```python
from build123d import *

# Parameters (mm, degrees)
SKETCH_R  = 1.05
SKETCH_W  = 12.4
SKETCH_H  = 23
PAD_DEPTH = 3
FILLET_R  = 4


with BuildPart() as part:
    # Sketch → Pad (new body)
    with BuildSketch(Plane.XY):
        Polygon((13, -50), (13, -74), (-13, -74), (-13, -50), (-13, -20), (-13, 12), (13, 12), (13, -20), align=None)
        with Locations((0, -41.76)):
            Circle(SKETCH_R, mode=Mode.SUBTRACT)
        with Locations((0, -69)):
            Circle(SKETCH_R, mode=Mode.SUBTRACT)
        with Locations((0, -55.38)):
            Rectangle(SKETCH_W, SKETCH_H, mode=Mode.SUBTRACT)
        with BuildLine():
            ThreePointArc((-6.5, 6), (-8, 7.5), (-9.5, 6))
            Line((-9.5, 6), (-9.5, -14))
            ThreePointArc((-9.5, -14), (-8, -15.5), (-6.5, -14))
            Line((-6.5, 6), (-6.5, -14))
        make_face(mode=Mode.SUBTRACT)
        with BuildLine():
            ThreePointArc((9.5, 6), (8, 7.5), (6.5, 6))
            Line((6.5, 6), (6.5, -14))
            ThreePointArc((6.5, -14), (8, -15.5), (9.5, -14))
            Line((9.5, 6), (9.5, -14))
        make_face(mode=Mode.SUBTRACT)
    extrude(amount=PAD_DEPTH)

    # Fillet
    fillet_edges = [part.edges().sort_by_distance(p)[0] for p in [
        (13, -74, 1.5),
        (-13, -74, 1.5),
        (13, 12, 1.5),
        (-13, 12, 1.5),
    ]]
    fillet(fillet_edges, radius=FILLET_R)


solid = part.part
```
Could you check a few things on this model? Use its own coordinates, in mm. A direction names the side the tool comes from. Give positions to 0.01 mm unless a question says otherwise; leave off trailing zeros. Loops run counter-clockwise (first coordinate to the right, second up) from the corner with the lowest first, then second, coordinate; pieces in that order, holes last. Notation, with made-up numbers: (85.5, -21) - (91.5, -21) arc R8 cw to (91.5, -10) - close; hole circle Ø4 at (59.25, 5). An arc over 180 degrees is marked (long way). Answer in a Markdown table with one row per item. Add a question column.
Q1. Which directions (+Z, -Z, +X, -X, +Y, -Y) give clear straight access to the entire face, cutting with the end or side of a thin tool? Please do faces 5 (the face through (-11.797, 10.859, 1.521)), 6 (the face through (8, 7.5, 1.5)).
Q2. If we section it at C-C (x = 5.25): List the corners of the cut face in (y, z) for me.
Q3. We'd pull the mould along Y, two halves only. Please class faces 1 (the face through (0, -74, 1)), 2 (the face through (0, -30, 0)), 3 (the face through (1, -68.68, 1.48)), 4 (the face through (11.859, 10.797, 1.521)): +Y half, -Y half, draft (parallel to the pull), parting line (faces both ways), or undercut.
Q4. If we section it at D-D (z = 1.25): List the corners of the cut face in (x, y) for me, plus the area to 3 significant figures.
Q5. Please list where these lines run through material, in increasing order: L1, parallel to Y at x = 0, z = 0.6; L2, parallel to X at y = -12, z = 2.35; L3, parallel to X at y = -65.5, z = 0.75. Write a range as from..to.
Q6. If we section it at A-A (y = -69): List the corners of the cut face in (x, z) for me, plus the area to 3 significant figures.
Q7. For pin 1 (1.3 mm diameter, centred on x = 0, y = -69, fed in from +Z) (3 decimals), with a flat end and sliding along its axis, tell me the tip position at first contact or that it passes through.
Q8. If we section it at B-B (y = 4): List the corners of the cut face in (x, z) for me.
The answers:
| question | item | result |
|---|---|---|
| 1 | face 5 | +Z, -Z, -X, +Y |
| 1 | face 6 | +Z, -Z |
| 2 | outline | (-74, 0) - (-66.88, 0) - (-66.88, 3) - (-74, 3) - close; (-43.88, 0) - (12, 0) - (12, 3) - (-43.88, 3) - close |
| 3 | face 1 | -Y half |
| 3 | face 2 | draft |
| 3 | face 3 | undercut |
| 3 | face 4 | +Y half |
| 4 | outline | (-13, -70) arc R4 ccw to (-9, -74) - (9, -74) arc R4 ccw to (13, -70) - (13, 8) arc R4 ccw to (9, 12) - (-9, 12) arc R4 ccw to (-13, 8) - close; hole (-9.5, -14) arc R1.5 ccw to (-6.5, -14) - (-6.5, 6) arc R1.5 ccw to (-9.5, 6) - close; hole (-6.2, -66.88) - (6.2, -66.88) - (6.2, -43.88) - (-6.2, -43.88) - close; hole circle Ø2.1 at (0, -69); hole circle Ø2.1 at (0, -41.76); hole (6.5, -14) arc R1.5 ccw to (9.5, -14) - (9.5, 6) arc R1.5 ccw to (6.5, 6) - close |
| 4 | area | 1,800 mm^2 |
| 5 | L1 | y = -74..-70.05, -67.95..-66.88, -43.88..-42.81, -40.71..12 |
| 5 | L2 | x = -13..-9.5, -6.5..6.5, 9.5..13 |
| 5 | L3 | x = -13..-6.2, 6.2..13 |
| 6 | outline | (-13, 0) - (-1.05, 0) - (-1.05, 3) - (-13, 3) - close; (1.05, 0) - (13, 0) - (13, 3) - (1.05, 3) - close |
| 6 | area | 71.7 mm^2 |
| 7 | pin 1 | passes through |
| 8 | outline | (-13, 0) - (-9.5, 0) - (-9.5, 3) - (-13, 3) - close; (-6.5, 0) - (6.5, 0) - (6.5, 3) - (-6.5, 3) - close; (9.5, 0) - (13, 0) - (13, 3) - (9.5, 3) - close |
